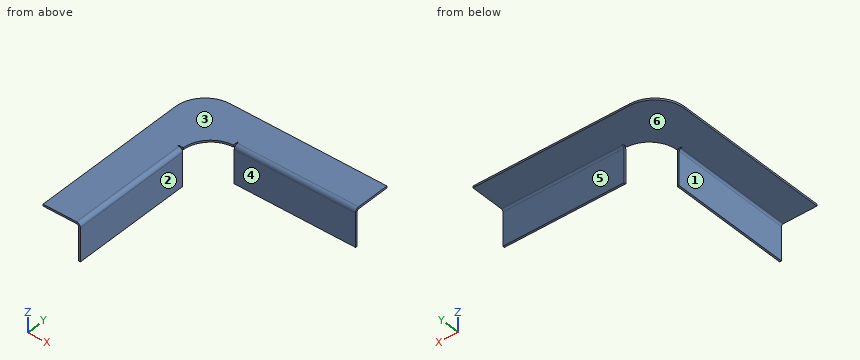
```python
from build123d import *

# Parameters (mm, degrees)
BASE_FLANGE1_DEPTH              = 1
EDGE_FLANGE1_STRIP_W            = 6
EDGE_FLANGE1_STRIP_H            = 1
EDGE_FLANGE1_STRIP_CUT_DEPTH    = 65
EDGE_FLANGE1_RELIEF_W           = 6.5
EDGE_FLANGE1_RELIEF_H           = 0.5
EDGE_FLANGE1_RELIEF_CUT_DEPTH   = 1
EDGE_FLANGE1_STRIP_2_W          = 6
EDGE_FLANGE1_STRIP_2_H          = 1
EDGE_FLANGE1_STRIP_CUT_2_DEPTH  = 65
EDGE_FLANGE1_RELIEF_2_W         = 6.5
EDGE_FLANGE1_RELIEF_2_H         = 0.5
EDGE_FLANGE1_RELIEF_CUT_2_DEPTH = 1
EDGE_FLANGE1_DEPTH              = 65
EDGE_FLANGE1_BEND_DEPTH         = 65


# Sheet-metal steps are written as plain solids
with BuildPart() as part:
    # Sketch1 → Base-Flange1 (new body)
    with BuildSketch(Plane.XY):
        with BuildLine():
            Line((-16, 0), (-16, -84))
            Line((-16, -84), (4, -84))
            Line((4, -84), (4, -19))
            ThreePointArc((4, -19), (8.393398282, -8.393398282), (19, -4))
            Line((19, -4), (84, -4))
            Line((84, -4), (84, 16))
            Line((84, 16), (0, 16))
            ThreePointArc((0, 16), (-11.313708499, 11.313708499), (-16, 0))
        make_face()
    extrude(amount=-BASE_FLANGE1_DEPTH)

    # Edge-Flange1 strip (across the edge) → Edge-Flange1 strip cut (cut)
    with BuildSketch(Plane(origin=(84, -4, -1), x_dir=(0, 1, 0), z_dir=(-1, 0, 0))):
        with Locations((-1, -0.5)):
            Rectangle(EDGE_FLANGE1_STRIP_W, EDGE_FLANGE1_STRIP_H)
    extrude(amount=EDGE_FLANGE1_STRIP_CUT_DEPTH, mode=Mode.SUBTRACT)

    # Edge-Flange1 relief (on the sheet) → Edge-Flange1 relief cut (cut)
    with BuildSketch(Plane(origin=(84, -2, -1), x_dir=(0, 1, 0), z_dir=(0, 0, -1))):
        with Locations((-2.75, -65.25)):
            Rectangle(EDGE_FLANGE1_RELIEF_W, EDGE_FLANGE1_RELIEF_H)
    extrude(amount=-EDGE_FLANGE1_RELIEF_CUT_DEPTH, mode=Mode.SUBTRACT)

    # Edge-Flange1 strip 2 (across the edge) → Edge-Flange1 strip cut 2 (cut)
    with BuildSketch(Plane(origin=(4, -19, -1), x_dir=(-1, 0, 0), z_dir=(0, -1, 0))):
        with Locations((-1, -0.5)):
            Rectangle(EDGE_FLANGE1_STRIP_2_W, EDGE_FLANGE1_STRIP_2_H)
    extrude(amount=EDGE_FLANGE1_STRIP_CUT_2_DEPTH, mode=Mode.SUBTRACT)

    # Edge-Flange1 relief 2 (on the sheet) → Edge-Flange1 relief cut 2 (cut)
    with BuildSketch(Plane(origin=(2, -19, -1), x_dir=(-1, 0, 0), z_dir=(0, 0, -1))):
        with Locations((-2.75, 0.25)):
            Rectangle(EDGE_FLANGE1_RELIEF_2_W, EDGE_FLANGE1_RELIEF_2_H)
    extrude(amount=-EDGE_FLANGE1_RELIEF_CUT_2_DEPTH, mode=Mode.SUBTRACT)

    # Edge-Flange1 section (across the edge) → Edge-Flange1 (add)
    with BuildSketch(Plane(origin=(84, -4, -1), x_dir=(0, 1, 0), z_dir=(-1, 0, 0))):
        with BuildLine():
            Line((0, 1), (0, 19))
            Line((0, 19), (1, 19))
            Line((1, 19), (1, 1))
            ThreePointArc((1, 1), (1.292893219, 0.292893219), (2, 0))
            Line((2, 0), (2, -1))
            ThreePointArc((2, -1), (0.585786438, -0.414213562), (0, 1))
        make_face()
    extrude(amount=EDGE_FLANGE1_DEPTH)

    # Edge-Flange1 section 2 (across the edge) → Edge-Flange1 bend (add)
    with BuildSketch(Plane(origin=(4, -19, -1), x_dir=(-1, 0, 0), z_dir=(0, -1, 0))):
        with BuildLine():
            Line((0, 1), (0, 19))
            Line((0, 19), (1, 19))
            Line((1, 19), (1, 1))
            ThreePointArc((1, 1), (1.292893219, 0.292893219), (2, 0))
            Line((2, 0), (2, -1))
            ThreePointArc((2, -1), (0.585786438, -0.414213562), (0, 1))
        make_face()
    extrude(amount=EDGE_FLANGE1_BEND_DEPTH)


solid = part.part
```
The listing builds one solid part. Answer for the finished solid, in the listing's coordinates (mm). Face numbers are marked on the shaded views. A direction names the side the tool comes from. Give positions to 0.01 mm unless a question says otherwise; leave off trailing zeros. Write each loop counter-clockwise with the first axis right and the second up, starting at its lowest first coordinate (ties: lowest second). Pieces come first, ordered by that corner, then holes. Notation, with made-up numbers: M 36.25,40 L 54.25,40 A14 ccw 54.25,54 Z; hole C -0.5,47 d10. An arc over 180 degrees is marked long. Write each question's results on one line, items separated by ' | '.
Q1. Section C-C, the plane x = 57.5 is taken. Write down the section's boundary in (y, z).
Output values:
outline: M -4,-20 L -3,-20 L -3,-2 A1 cw -2,-1 L 16,-1 L 16,0 L -2,0 A2 ccw -4,-2 Z
Q2. Section A-A, the plane z = -17.25 is taken. Write down the section's boundary in (x, y), then the cut area to 3 significant figures.
Output values:
outline: M 3,-84 L 4,-84 L 4,-19 L 3,-19 Z; M 19,-4 L 84,-4 L 84,-3 L 19,-3 Z | area: 130 mm2
Q3. Flat-ended cylindrical pins translate along their axes: P1, Ø1, axis at y = -28, z = -2.5, coming from the -X side; P2, Ø0.6, axis at y = -18.5, z = -0.5, coming from the +X side; P3, Ø12, axis at x = 41, y = -2.5, coming from the +Z side; P4, Ø3, axis at y = -2, z = -7.5, coming from the -X side. Find the tip coordinate at first contact, or state that the pin passes through.
Output values:
P1: x = 3 | P2: x = 4.02 | P3: z = 0 | P4: x = 19
Q4. Section B-B, the plane y = -54 is taken. Write down the section's boundary in (x, z).
Output values:
outline: M -16,-1 L 2,-1 A1 cw 3,-2 L 3,-20 L 4,-20 L 4,-2 A2 ccw 2,0 L -16,0 Z
Q5. A tool of negligible diameter and unlimited length cuts with its end or side. For the marked faces 4, 5 and 6, from which of +Z, -Z, +X, -X, +Y, -Y can it reach the whole face along a straight path? Write none if from no direction.
Output values:
face 4: +Z, -Z, +X, -X, -Y | face 5: -Z, +X, -X, +Y | face 6: -Z, -X, +Y
Q6. Consider L1, parallel to X at y = -77, z = -16.75; L2, parallel to Y at x = 60, z = -9.25; L3, parallel to Z at x = 0, y = -5.5. Determine where each line is inside the solid, lowest interval first. Write a range as from..to.
Output values:
L1: 3..4 | L2: -4..-3 | L3: -1..0
Q7. For a pull along X with two mould halves and no side action, classify the marked faces 1, 2 and 3 as released by +X, released by -X, zero draft, split by the parting line, or undercut.
Output values:
face 1: released by -X | face 2: released by +X | face 3: zero draft
Q8. Section D-D, the plane x = 10 is taken. Write down the section's boundary in (y, z).
Output values:
outline: M -7,-1 L 16,-1 L 16,0 L -7,0 Z
